For this review, take the finished solid that the model builds, in its own axes (mm). Face numbers are marked on the shaded views. A direction names the side the tool comes from. Coordinates: 2 decimals unless noted, no trailing zeros. Loops run counter-clockwise (first coordinate to the right, second up) from the corner with the lowest first, then second, coordinate; pieces in that order, holes last. Notation, with made-up numbers: M -7,0.25 L 27,0.25 A21 cw 27,24.25 Z; hole C -4.5,39.25 d3. An arc over 180 degrees is marked long. Answer as a JSON object with one key per item and string values. Group by question number.
Item 1: Wall thickness on L1, parallel to X at y = 47.5, z = 1; L2, parallel to Z at x = -2.75, y = 32; L3, parallel to Z at x = -1.75, y = 46: over which ranges is each line inside the solid? List them lowest first. Write a range as from..to.
Item 2: Add section A-A (z = 0). State the section outline as (x, y) points, then the cut area to 3 significant figures.
Item 3: Mouldability with a two-part tool opening along X and no side actions: class the marked faces 1, 2, 3 and 4 as +X half, -X half, draft (parallel to the pull), parting line (faces both ways), or undercut.
Item 4: Tool access review of the marked faces 5 and 6: name each direction out of +Z, -Z, +X, -X, +Y, -Y from which nothing blocks a thin tool from reaching the whole face with its end or side.
Item 5: Insertion check: pin 1 (3 mm diameter, centred on x = -4, z = 0, fed in from +Y); pin 2 (1.5 mm diameter, centred on x = -0.5, y = 31.5, fed in from -Z); pin 3 (3 mm diameter, centred on y = 36, z = 8, fed in from +X). Each pin has a flat end and moves straight along its axis. Give the tip position at first contact, or say it passes through.
Item 6: Add section B-B (x = 4). State the section outline as (y, z) points (3 decimals).
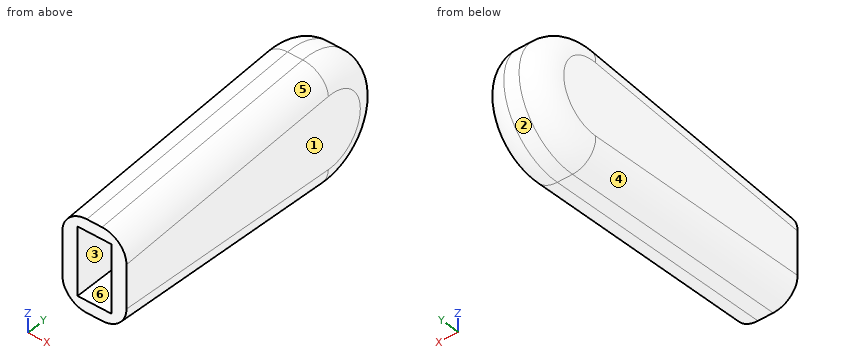
Autodesk Inventor part; units mm, degrees
ref_plane "YZ Plane" through (0, 0, 0) normal (1, 0, 0) x (0, 1, 0)
ref_plane "XZ Plane" through (0, 0, 0) normal (0, 1, 0) x (-1, 0, 0)
ref_plane "XY Plane" through (0, 0, 0) normal (0, 0, 1) x (1, 0, 0)
sketch "Sketch1" plane through (0, 0, 0) normal (1, 0, 0) x (0, 1, 0)
  line L0 (47.76, 6.35) -> (1.01, 6.35)
  arc A0 (47.76, -6.35) -> (47.76, 6.35) centre (47.76, 0) ccw
  line L1 (1.01, -6.35) -> (47.76, -6.35)
  arc A1 (45.5521, -11.1807) -> (45.5521, 11.1807) centre (46.21, 0) ccw
  line L2 (1.01, 8.56) -> (45.5521, 11.1807)
  line L3 (1.01, -8.56) -> (45.5521, -11.1807)
  line L4 (1.01, 8.56) -> (1.01, -8.56)
  point P0 (0.24, 0)
  point P1 (1.01, 0)
  point P2 (0, 0)
  dimension "d0" = 17.12
  dimension "d2" = 11.2
  dimension "d3" = 2.21
  dimension "d4" = 46.75
  dimension "d5" = 45.2
  dimension "d7" = 8.5
  dimension "d9" = 0.24
extrude "Extrusion1" add sketch "Sketch1" along normal mid plane 11.8
fillet "Fillet1" radius 4.5 6 edges at (5.9, 57.41, 0) (5.9, 23.281, 9.8703) (5.9, 23.281, -9.8703) (-5.9, 57.41, 0) (-5.9, 23.281, 9.8703) (-5.9, 23.281, -9.8703)
extrude "Extrusion2" cut sketch "Sketch1" along normal mid plane 6.2 contours A0 L1 L4 L0
properties part number "Grip_1"
From the geometry:
{
 "1": {"L1": "x = -5.9..-3.1, 3.1..5.9", "L2": "z = -10.18..-6.35, 6.35..10.18", "L3": "z = -11.18..-6.35, 6.35..11.18"},
 "2": {"outline": "M -5.9,1.01 L -3.1,1.01 L -3.1,54.11 L 3.1,54.11 L 3.1,1.01 L 5.9,1.01 L 5.9,52.91 A4.5 ccw 1.4,57.41 L -1.4,57.41 A4.5 ccw -5.9,52.91 Z", "area": "328 mm²"},
 "3": {"face 1": "+X half", "face 2": "draft", "face 3": "undercut", "face 4": "-X half"},
 "4": {"face 5": "+Z, +X, -Y", "face 6": "-Y"},
 "5": {"pin 1": "stops at y = 57.27", "pin 2": "stops at z = -10.4", "pin 3": "stops at x = 5.88"},
 "6": {"outline": "M 1.01,-7.731 L 45.601,-10.355 A10.373 ccw long 45.601,10.355 L 1.01,7.731 Z"}
}
